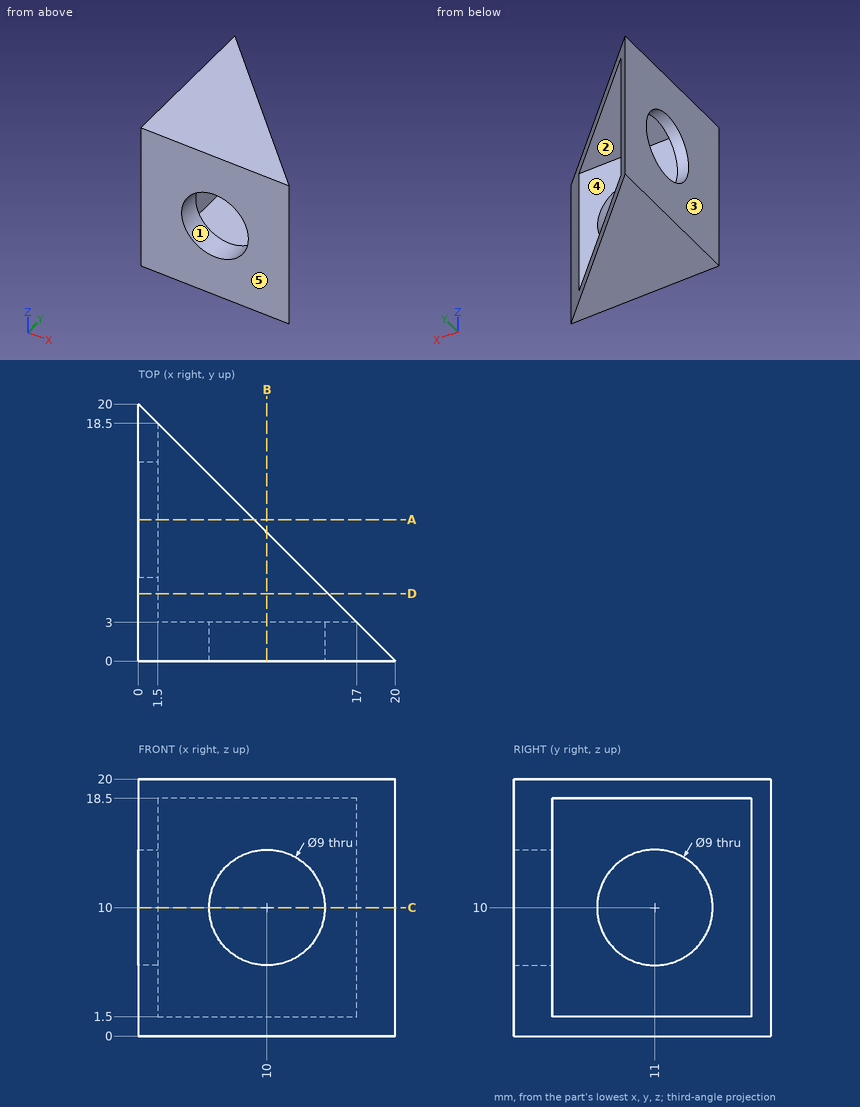
Geometry: see drawing. Coordinates: mm, zero at the bounding-box minimum. A direction names the side the tool comes from. Coordinates: 2 decimals unless noted, no trailing zeros. Order: outer loops, then holes, each group sorted by start corner. A loop starts at its lowest first (then second) coordinate and runs counter-clockwise, first axis right, second up. Notation, with made-up numbers: (86.5, -39.5) - (136.5, -39.5) arc R17 cw to (136.5, -6.5) - close; hole circle Ø6 at (-1.75, 77.5). An arc over 180 degrees is marked (long way). Use one line per item in the form item = value.
1) Section A-A (y = 11). Return loops of the section in (x, z).
Solutions:
outline = (0, 0) - (9, 0) - (9, 1.5) - (1.5, 1.5) - (1.5, 5.5) - (0, 5.5) - close; (0, 14.5) - (1.5, 14.5) - (1.5, 18.5) - (9, 18.5) - (9, 20) - (0, 20) - close
2) Pin query (flat end, axial travel): pin 1 (4.5 mm diameter, centred on y = 9.5, z = 6.5, fed in from +X); pin 2 (8 mm diameter, centred on x = 14.5, z = 6, fed in from +Y). Return the tip coordinate at first contact, or that it passes through.
Solutions:
pin_1 = 1.5
pin_2 = 3
3) Section D-D (y = 5.25). Return loops of the section in (x, z), then the cut area to 4 significant figures.
Solutions:
outline = (0, 0) - (14.75, 0) - (14.75, 1.5) - (1.5, 1.5) - (1.5, 18.5) - (14.75, 18.5) - (14.75, 20) - (0, 20) - close
area = 69.75 mm^2
4) Set-up query: the marked faces 4 and 5. Return all of +Z, -Z, +X, -X, +Y, -Y with unobstructed straight access to the full face (end or side cutting, diameter ignored); none if empty.
Solutions:
face_4 = +X, +Y
face_5 = +Z, -Z, +X, -X, -Y
5) Mould query, pull axis X, two halves, no side actions, for the marked faces 1, 2 and 3. Classes: +X half, -X half, draft (parallel to the pull), parting line (faces both ways), or undercut.
Solutions:
face_1 = undercut
face_2 = draft
face_3 = -X half
6) Ray query, L1, parallel to Z at x = 10, y = 0.75; L2, parallel to Z at x = 6, y = 10.25; L3, parallel to Y at x = 8.75, z = 4.75. Return the intervals inside material, ascending.
Solutions:
L1 = 0 to 5.5, 14.5 to 20
L2 = 0 to 1.5, 18.5 to 20
L3 = 0 to 3
7) Section B-B (x = 10). Return loops of the section in (y, z).
Solutions:
outline = (0, 0) - (10, 0) - (10, 1.5) - (3, 1.5) - (3, 5.5) - (0, 5.5) - close; (0, 14.5) - (3, 14.5) - (3, 18.5) - (10, 18.5) - (10, 20) - (0, 20) - close
8) Section C-C (z = 10). Return loops of the section in (x, y).
Solutions:
outline = (0, 0) - (5.5, 0) - (5.5, 3) - (1.5, 3) - (1.5, 6.5) - (0, 6.5) - close; (0, 15.5) - (1.5, 15.5) - (1.5, 18.5) - (0, 20) - close; (14.5, 0) - (20, 0) - (17, 3) - (14.5, 3) - close
